For this review, take the finished solid that the model builds, in its own axes (mm). A direction names the side the tool comes from. Coordinates: 2 decimals unless noted, no trailing zeros. Loops run counter-clockwise (first coordinate to the right, second up) from the corner with the lowest first, then second, coordinate; pieces in that order, holes last. Notation, with made-up numbers: M -7,-7.5 L 0,-7.5 A20 cw 0,25.5 Z; hole C -28,32.5 d3. An arc over 180 degrees is marked long. Answer as a JSON object with one key per item and string values. Group by question number.
Item 1: Add section C-C (y = -55.5). State the section outline as (x, z) points.
Item 2: Wall thickness on L1, parallel to Z at x = 0.05, y = -15; L2, parallel to Y at x = 0.8, z = 3 (3 decimals); L3, parallel to Y at x = -0.5, z = -6 (1 decimal): over which ranges is each line inside the solid? List them lowest first. Write a range as from..to.
Item 3: Tool access review of faces 1 (the face through (1.206, -55, 1)), 2 (the face through (0, -56, -0.039)): name each direction out of +Z, -Z, +X, -X, +Y, -Y from which nothing blocks a thin tool from reaching the whole face with its end or side.
Item 4: Add section A-A (z = -11). State the section outline as (x, y) points (3 decimals), then the cut area to 3 significant figures.
Item 5: Add section B-B (x = 0.55). State the section outline as (y, z) points (3 decimals), then the cut area to 3 significant figures.
Item 6: Mouldability with a two-part tool opening along Y and no side actions: class faces 3 (the face through (0, -56, 15)), 4 (the face through (0, -10.795, -10)), 5 (the face through (0.22, -51.128, -0.505)), 6 (the face through (0, -100.745, -10)) as +Y half, -Y half, draft (parallel to the pull), parting line (faces both ways), or undercut.
Item 7: Add section D-D (z = -17). State the section outline as (x, y) points (3 decimals).
from build123d import *

# Parameters (mm, degrees)
EXTRUDE_1_DEPTH     = 2
FILLET_1_R          = 2
FILLET_2_R          = 2
FILLET_3_R          = 2
FILLET_4_R          = 2
SKETCH_2_W          = 12
SKETCH_2_H          = 89.95
EXTRUDE_2_DEPTH     = 2
CUT_EXTRUDE_1_DEPTH = 10
SKETCH_7_R          = 1.6
CUT_EXTRUDE_2_DEPTH = 10
SKETCH_8_W          = 10
SKETCH_8_H          = 28.446825321
EXTRUDE_3_DEPTH     = 2


with BuildPart() as part:
    # 草图1 → 凸台-拉伸1 (new body)
    with BuildSketch(Plane(origin=(-0.79375, 0, 0), x_dir=(0, -1, 0), z_dir=(-1, 0, 0))):
        with BuildLine():
            Line((38.795, 5), (12.795, 5))
            ThreePointArc((12.795, 5), (11.380786438, 4.414213562), (10.795, 3))
            Line((10.795, 3), (10.795, -13))
            ThreePointArc((10.795, -13), (11.380786438, -14.414213562), (12.795, -15))
            Line((12.795, -15), (47.795, -15))
            Line((47.795, -15), (50.77, -0.039144756))
            Line((50.77, -0.039144756), (55.77, -0.039144756))
            Line((55.77, -0.039144756), (60.77, -0.039144756))
            Line((60.77, -0.039144756), (63.745, -15))
            Line((63.745, -15), (98.745, -15))
            ThreePointArc((98.745, -15), (100.159213562, -14.414213562), (100.745, -13))
            Line((100.745, -13), (100.745, 3))
            ThreePointArc((100.745, 3), (100.159213562, 4.414213562), (98.745, 5))
            Line((98.745, 5), (72.745, 5))
            Line((72.745, 5), (38.795, 5))
        make_face()
    extrude(amount=-EXTRUDE_1_DEPTH)

    # 圆角1
    fillet_1_edges = [part.edges().sort_by_distance(p)[0] for p in [
        (0.20625, -50.77, -0.039144756),
    ]]
    fillet(fillet_1_edges, radius=FILLET_1_R)

    # 圆角2
    fillet_2_edges = [part.edges().sort_by_distance(p)[0] for p in [
        (0.20625, -47.795, -15),
    ]]
    fillet(fillet_2_edges, radius=FILLET_2_R)

    # 圆角3
    fillet_3_edges = [part.edges().sort_by_distance(p)[0] for p in [
        (0.20625, -60.77, -0.039144756),
    ]]
    fillet(fillet_3_edges, radius=FILLET_3_R)

    # 圆角4
    fillet_4_edges = [part.edges().sort_by_distance(p)[0] for p in [
        (0.20625, -63.745, -15),
    ]]
    fillet(fillet_4_edges, radius=FILLET_4_R)

    # 草图2 → 凸台-拉伸2 (add)
    with BuildSketch(Plane.ZY.offset(0.79375)):
        with Locations((9, -55.77)):
            Rectangle(SKETCH_2_W, SKETCH_2_H)
        Polygon((-25, -10.795), (-25, -45.806477318), (-13.39006724, -48.115138781), (-13, -10.795), align=None)
        Polygon((-13.39006724, -63.424861219), (-25, -65.733522682), (-25, -100.745), (-13, -100.745), align=None)
    extrude(amount=-EXTRUDE_2_DEPTH)

    # 草图5 → 切除-拉伸1 (cut)
    with BuildSketch(Plane(origin=(1.20625, 0, 0), x_dir=(0, 0, -1), z_dir=(1, 0, 0))):
        Polygon((1.649077515, -50.449861219), (25, -45.806477318), (25, -39.241825321), align=None)
        Polygon((25, -72.298174679), (25, -65.733522682), (1.649077515, -61.090138781), align=None)
    extrude(amount=-CUT_EXTRUDE_1_DEPTH, mode=Mode.SUBTRACT)

    # 草图7 → 切除-拉伸2 (cut)
    with BuildSketch(Plane(origin=(1.20625, 0, 0), x_dir=(0, 0, -1), z_dir=(1, 0, 0))):
        with Locations((-2.960855244, -14.795)):
            Circle(SKETCH_7_R)
        with Locations((3.039144756, -14.795)):
            Circle(SKETCH_7_R)
        with Locations((3.039144756, -96.745)):
            Circle(SKETCH_7_R)
        with Locations((-2.960855244, -96.745)):
            Circle(SKETCH_7_R)
    extrude(amount=-CUT_EXTRUDE_2_DEPTH, mode=Mode.SUBTRACT)

    # 草图8 → 凸台-拉伸3 (add)
    with BuildSketch(Plane.ZY.offset(0.79375)):
        with Locations((-30, -25.018412661)):
            Rectangle(SKETCH_8_W, SKETCH_8_H)
        with Locations((-30, -86.52158734)):
            Rectangle(SKETCH_8_W, SKETCH_8_H)
    extrude(amount=-EXTRUDE_3_DEPTH)


solid = part.part
From the geometry:
{
 "1": {"outline": "M -0.79,-0.04 L 1.21,-0.04 L 1.21,15 L -0.79,15 Z"},
 "2": {"L1": "z = -35..-4.63, -1.45..1.37, 4.55..15", "L2": "y = -100.745..-98.345, -95.145..-16.395, -13.195..-10.795", "L3": "y = -100.7..-63.2, -48.4..-10.8"},
 "3": {"face 1": "+Z, -Z, +X, +Y, -Y", "face 2": "-Z, +X, -X"},
 "4": {"outline": "M -0.794,-100.745 L 1.206,-100.745 L 1.206,-65.578 L -0.794,-65.578 Z; M -0.794,-45.962 L 1.206,-45.962 L 1.206,-10.795 L -0.794,-10.795 Z", "area": "141 mm²"},
 "5": {"outline": "M -100.745,-35 L -72.298,-35 L -72.298,-25 L -61.09,-1.649 A2 cw -59.129,-0.039 L -52.411,-0.039 A2 cw -50.45,-1.649 L -39.242,-25 L -39.242,-35 L -10.795,-35 L -10.795,15 L -100.745,15 Z; hole C -96.745,-3.039 d3.2; hole C -96.745,2.961 d3.2; hole C -14.795,-3.039 d3.2; hole C -14.795,2.961 d3.2", "area": "3,610 mm²"},
 "6": {"face 3": "draft", "face 4": "+Y half", "face 5": "undercut", "face 6": "-Y half"},
 "7": {"outline": "M -0.794,-100.745 L 1.206,-100.745 L 1.206,-68.458 L -0.794,-68.458 Z; M -0.794,-43.082 L 1.206,-43.082 L 1.206,-10.795 L -0.794,-10.795 Z"}
}
